Geometry check sheet. Reference: the model listing, model coordinates, mm. A direction names the side the tool comes from. Coordinates: 2 decimals unless noted, no trailing zeros. Loops run counter-clockwise (first coordinate to the right, second up) from the corner with the lowest first, then second, coordinate; pieces in that order, holes last.
from build123d import *

# Parameters (mm, degrees)
F1_DEPTH       = 158.75
F3_DEPTH       = 6.351
F5_D           = 6.5278
F5_CSINK_D     = 13.4874
F5_CSINK_ANGLE = 82
F6_R           = 3.175


with BuildPart() as f1:
    # F0 (on Right) → F1 (new body)
    with BuildSketch(Plane.YZ):
        Polygon((20.6375, 20.6375), (14.2875, 20.6375), (14.2875, -14.2875), (-20.6375, -14.2875), (-20.6375, -20.6375), (20.6375, -20.6375), align=None)
    extrude(amount=F1_DEPTH)

    # F2 (on face) → F3 (cut, through all)
    with BuildSketch(Plane.XZ.offset(-14.2875)):
        with BuildLine():
            ThreePointArc((19.05, 8.9789), (15.0876, 5.0165), (19.05, 1.0541))
            Line((19.05, 1.0541), (139.7, 1.0541))
            ThreePointArc((139.7, 1.0541), (143.6624, 5.0165), (139.7, 8.9789))
            Line((139.7, 8.9789), (19.05, 8.9789))
        make_face()
    extrude(amount=-F3_DEPTH, mode=Mode.SUBTRACT)

    # F5 (through all)
    with Locations(Plane.XY.offset(-14.2875)):
        with Locations((15.875, -1.5875), (142.875, -1.5875)):
            CounterSinkHole(F5_D / 2, F5_CSINK_D / 2, counter_sink_angle=F5_CSINK_ANGLE)

    # F6
    f6_edges = [f1.edges().sort_by_distance(p)[0] for p in [
        (0, 17.4625, 20.6375),
        (158.75, 17.4625, 20.6375),
        (158.75, -20.6375, -17.4625),
        (0, -20.6375, -17.4625),
    ]]
    fillet(f6_edges, radius=F6_R)


solid = f1.part
1) Section check D-D on z = 11. Record the cut outline in (x, y), and give its area (3 significant figures).
Data:
outline: (0, 14.29) - (158.75, 14.29) - (158.75, 20.64) - (0, 20.64) - close
area: 1,010 mm2
2) Mould release check, pull along Z, two halves, no side actions. Record for faces 4 (the flat face through (78, -3, -14.288)), 5 (the cylindrical face through (143.66, 17.42, 4.93)), 6 (the cylindrical face through (0.95, -19.73, -17.51)): +Z half, -Z half, draft (parallel to the pull), parting line (faces both ways), or undercut.
Data:
face 4: +Z half
face 5: undercut
face 6: draft
3) Section check C-C on z = 5. Record the cut outline in (x, y).
Data:
outline: (0, 14.29) - (15.09, 14.29) - (15.09, 20.64) - (0, 20.64) - close; (143.66, 14.29) - (158.75, 14.29) - (158.75, 20.64) - (143.66, 20.64) - close
4) Access from +Z, -Z, +X, -X, +Y, -Y to the whole of each face (thin tool, end or side, straight path). Record for faces 1 (the flat face through (78, 14.288, 0)), 2 (the cylindrical face through (0.95, 17.42, 19.73)), 3 (the flat face through (79, 17, 1.054)).
Data:
face 1: +Z, +X, -X, -Y
face 2: +Z, -X, +Y, -Y
face 3: +Y, -Y
5) Section check A-A on x = 74. Record the cut outline in (y, z).
Data:
outline: (-20.64, -20.64) - (20.64, -20.64) - (20.64, 1.05) - (14.29, 1.05) - (14.29, -14.29) - (-20.64, -14.29) - close; (14.29, 8.98) - (20.64, 8.98) - (20.64, 20.64) - (14.29, 20.64) - close
6) Material ranges on probe 1 along Z at (x, y) = (68, -2.5); probe 2 along Y at (x, z) = (94, -5); probe 3 along Z at (x, y) = (19, -4.5), recorded low to high.
Data:
probe 1: z = -20.64 to -14.29
probe 2: y = 14.29 to 20.64
probe 3: z = -20.64 to -17.13
7) Depth check by flat-ended pin: pin 1 (17.5 mm diameter, centred on x = 59.5, z = 5.5, fed in from -Y); pin 2 (1 mm diameter, centred on x = 34.5, y = 2, fed in from +Z). Enter the tip coordinate at first touch or a pass-through.
Data:
pin 1: stops at y = 14.29
pin 2: stops at z = -14.29
